Autodesk Inventor part; units mm, degrees
ref_plane "YZ Plane" through (0, 0, 0) normal (1, 0, 0) x (0, 1, 0)
ref_plane "XZ Plane" through (0, 0, 0) normal (0, 1, 0) x (-1, 0, 0)
ref_plane "XY Plane" through (0, 0, 0) normal (0, 0, 1) x (1, 0, 0)
sketch "Boceto6" plane through (0, 0, 0) normal (0, 1, 0) x (-1, 0, 0)
  line L0 (0, 0) -> (100, 0)
  line L1 (100, 0) -> (100, -100)
  line L2 (100, -100) -> (0, -100)
  line L3 (0, -100) -> (0, 0)
  line L4 (97, -97) -> (97, -3)
  line L5 (97, -3) -> (3, -3)
  line L6 (3, -3) -> (3, -97)
  line L7 (3, -97) -> (97, -97)
  line L8 (97, -3) -> (100, -3)
  line L9 (3, -97) -> (3, -106.6251)
  point P0 (3, -100)
  dimension "d46" = 100
  dimension "d47" = 100
  dimension "d48" = 3
extrude "Extrusión6" add sketch "Boceto6" along normal blind 2000 contours L0 L1 L8 L5 L6 L9 L2 L3
sketch "Boceto9" plane through (-100, 0, 0) normal (0, 0, 1) x (1, 0, 0)
  point P0 (100, 0)
sketch "Boceto12" plane through (0, 0, 0) normal (1, 0, 0) x (0, 0, -1)
  line L0 (0, 2000) -> (100, 2000)
  line L1 (100, 0) -> (100, 2000)
  line L2 (0, 2000) -> (100, 2000)
  line L3 (100, 2000) -> (100, 1950)
  line L4 (100, 1950) -> (0, 1950)
  line L5 (0, 1950) -> (0, 2000)
  line L6 (0, 1650) -> (100, 1650)
  line L7 (100, 1650) -> (100, 1600)
  line L8 (100, 1600) -> (0, 1600)
  line L9 (0, 1600) -> (0, 1650)
  line L10 (0, 1300) -> (100, 1300)
  line L11 (100, 1300) -> (100, 1250)
  line L12 (100, 1250) -> (0, 1250)
  line L13 (0, 1250) -> (0, 1300)
  line L14 (0, 950) -> (100, 950)
  line L15 (100, 950) -> (100, 900)
  line L16 (100, 900) -> (0, 900)
  line L17 (0, 900) -> (0, 950)
  line L18 (0, 600) -> (100, 600)
  line L19 (100, 600) -> (100, 550)
  line L20 (100, 550) -> (0, 550)
  line L21 (0, 550) -> (0, 600)
  circle A0 centre (50, 1900) radius 25
  line L22 (0, 0) -> (0, 2000)
  circle A1 centre (50, 1800) radius 25
  circle A2 centre (50, 1700) radius 25
  circle A3 centre (20, 1975) radius 4
  circle A4 centre (45, 1975) radius 4
  circle A5 centre (70, 1975) radius 4
  line L23 (100, 1600) -> (0, 1600)
  line L24 (0, 1650) -> (100, 1650)
  line L25 (100, 1650) -> (100, 1600)
  circle A6 centre (50, 1350) radius 25
  circle A7 centre (50, 1450) radius 25
  circle A8 centre (50, 1550) radius 25
  circle A9 centre (70, 1625) radius 4
  circle A10 centre (45, 1625) radius 4
  circle A11 centre (20, 1625) radius 4
  line L26 (100, 1250) -> (0, 1250)
  line L27 (0, 1300) -> (100, 1300)
  line L28 (100, 1300) -> (100, 1250)
  circle A12 centre (50, 1000) radius 25
  circle A13 centre (50, 1100) radius 25
  circle A14 centre (50, 1200) radius 25
  circle A15 centre (70, 1275) radius 4
  circle A16 centre (45, 1275) radius 4
  circle A17 centre (20, 1275) radius 4
  line L29 (100, 900) -> (0, 900)
  line L30 (0, 950) -> (100, 950)
  line L31 (100, 950) -> (100, 900)
  circle A18 centre (50, 650) radius 25
  circle A19 centre (50, 750) radius 25
  circle A20 centre (50, 850) radius 25
  circle A21 centre (70, 925) radius 4
  circle A22 centre (45, 925) radius 4
  circle A23 centre (20, 925) radius 4
  line L32 (100, 550) -> (0, 550)
  line L33 (0, 600) -> (100, 600)
  line L34 (100, 600) -> (100, 550)
  circle A24 centre (50, 300) radius 25
  circle A25 centre (50, 400) radius 25
  circle A26 centre (50, 500) radius 25
  circle A27 centre (70, 575) radius 4
  circle A28 centre (45, 575) radius 4
  circle A29 centre (20, 575) radius 4
  point P0 (0, 1975)
  point P1 (100, 1975)
  point P2 (100, 1625)
  point P3 (100, 1275)
  point P4 (100, 925)
  point P5 (100, 575)
  dimension "d113" = 50
  dimension "d116" = 350
  dimension "d121" = 50
  dimension "d122" = 50
  dimension "d123" = 50
  dimension "d126" = 100
  dimension "d135" = 8
  dimension "d136" = 8
  dimension "d137" = 8
  dimension "d138" = 25
  dimension "d139" = 25
  dimension "d140" = 25
  dimension "d141" = 20
  dimension "d142" = 30
  dimension "d143" = 25
  dimension "d144" = 25
  dimension "d147" = 350
extrude "Extrusión10" cut sketch "Boceto12" against normal blind 2000 contours A0 | A1 | A2 | A3 | A4 | A5 | A6 | A7 | A8 | A9 | A10 | A11 | A12 | A13 | A14 | A15 | A16 | A17 | A18 | A19 | A20 | A21 | A22 | A23 | A24 | A25 | A26 | A27 | A28 | A29
sketch "Boceto13" plane through (-100, 0, 0) normal (0, 0, 1) x (1, 0, 0)
  line L0 (0, 2000) -> (100, 2000)
  line L1 (100, 694.7481) -> (100, 2000)
  line L2 (0, 2000) -> (100, 2000)
  line L3 (100, 2000) -> (100, 1950)
  line L4 (100, 1950) -> (0, 1950)
  line L5 (0, 1950) -> (0, 2000)
  line L6 (0, 1650) -> (100, 1650)
  line L7 (100, 1650) -> (100, 1600)
  line L8 (100, 1600) -> (0, 1600)
  line L9 (0, 1600) -> (0, 1650)
  line L10 (0, 1300) -> (100, 1300)
  line L11 (100, 1300) -> (100, 1250)
  line L12 (100, 1250) -> (0, 1250)
  line L13 (0, 1250) -> (0, 1300)
  line L14 (0, 950) -> (100, 950)
  line L15 (100, 950) -> (100, 900)
  line L16 (100, 900) -> (0, 900)
  line L17 (0, 900) -> (0, 950)
  line L18 (0, 600) -> (100, 600)
  line L19 (100, 600) -> (100, 550)
  line L20 (100, 550) -> (0, 550)
  line L21 (0, 550) -> (0, 600)
  circle A0 centre (50, 1900) radius 25
  line L22 (0, 692.1927) -> (0, 2000)
  circle A1 centre (50, 1800) radius 25
  circle A2 centre (50, 1700) radius 25
  circle A3 centre (20, 1975) radius 4
  circle A4 centre (45, 1975) radius 4
  circle A5 centre (70, 1975) radius 4
  line L23 (100, 1600) -> (0, 1600)
  line L24 (0, 1650) -> (100, 1650)
  line L25 (100, 1650) -> (100, 1600)
  circle A6 centre (50, 1350) radius 25
  circle A7 centre (50, 1450) radius 25
  circle A8 centre (50, 1550) radius 25
  circle A9 centre (70, 1625) radius 4
  circle A10 centre (45, 1625) radius 4
  circle A11 centre (20, 1625) radius 4
  line L26 (100, 1250) -> (0, 1250)
  line L27 (0, 1300) -> (100, 1300)
  line L28 (100, 1300) -> (100, 1250)
  circle A12 centre (50, 1000) radius 25
  circle A13 centre (50, 1100) radius 25
  circle A14 centre (50, 1200) radius 25
  circle A15 centre (70, 1275) radius 4
  circle A16 centre (45, 1275) radius 4
  circle A17 centre (20, 1275) radius 4
  line L29 (100, 900) -> (0, 900)
  line L30 (0, 950) -> (100, 950)
  line L31 (100, 950) -> (100, 900)
  circle A18 centre (50, 650) radius 25
  circle A19 centre (50, 750) radius 25
  circle A20 centre (50, 850) radius 25
  circle A21 centre (70, 925) radius 4
  circle A22 centre (45, 925) radius 4
  circle A23 centre (20, 925) radius 4
  line L32 (100, 550) -> (0, 550)
  line L33 (0, 600) -> (100, 600)
  line L34 (100, 600) -> (100, 550)
  circle A24 centre (50, 300) radius 25
  circle A25 centre (50, 400) radius 25
  circle A26 centre (50, 500) radius 25
  circle A27 centre (70, 575) radius 4
  circle A28 centre (45, 575) radius 4
  circle A29 centre (20, 575) radius 4
  line L35 (0, 0) -> (0, 2000)
  line L36 (100, 0) -> (100, 2000)
  line L37 (0, 2000) -> (100, 2000)
  point P0 (0, 1975)
  point P1 (100, 1975)
  point P2 (100, 1625)
  point P3 (100, 1275)
  point P4 (100, 925)
  point P5 (100, 575)
  dimension "d166" = 50
  dimension "d167" = 350
  dimension "d168" = 50
  dimension "d169" = 50
  dimension "d170" = 50
  dimension "d171" = 100
  dimension "d172" = 8
  dimension "d173" = 8
  dimension "d174" = 8
  dimension "d175" = 25
  dimension "d176" = 25
  dimension "d177" = 25
  dimension "d178" = 20
  dimension "d179" = 30
  dimension "d180" = 25
  dimension "d181" = 25
  dimension "d182" = 350
  dimension "d186" = 0
  dimension "d187" = 0
  dimension "d188" = 0
extrude "Extrusión11" cut sketch "Boceto13" against normal blind 2000 contours A0 | A1 | A2 | A3 | A4 | A5 | A6 | A7 | A8 | A9 | A10 | A11 | A12 | A13 | A14 | A15 | A16 | A17 | A18 | A19 | A20 | A21 | A22 | A23 | A24 | A25 | A26 | A27 | A28 | A29
properties part number "mesa completa"
Source: CAD feature listing. Evaluate the final solid. Frame: model axes, mm. Round coordinates to 2 decimals unless told otherwise and drop trailing zeros. Loops run counter-clockwise (first coordinate to the right, second up) from the corner with the lowest first, then second, coordinate; pieces in that order, holes last.
(1) Material intervals for probe 1 along X at (y, z) = (1625, -2); probe 2 along Z at (x, y) = (-0.55, 925); probe 3 along X at (y, z) = (1350, -2.3), sorted ascending.
From the geometry:
probe 1: x = -100 to -84, -76 to -59, -51 to -34, -26 to 0
probe 2: z = -100 to -74, -66 to -49, -41 to -24, -16 to 0
probe 3: x = -100 to -75, -25 to 0
(2) Contact query for flat-ended pins moving along their axis: pin 1 Ø10.5 at (x, y) = (-80, 575) entering from -Z; pin 2 Ø5 at (y, z) = (537, -30.5) entering from -X. Output: stop coordinate, or through.
From the geometry:
pin 1: stops at z = -3
pin 2: stops at x = -3
(3) Section query A-A (y = 1800). Output: boundary loops of the cut face in (x, z).
From the geometry:
outline: (-100, -3) - (-75, -3) - (-75, 0) - (-100, 0) - close; (-25, -3) - (-3, -3) - (-3, -25) - (0, -25) - (0, 0) - (-25, 0) - close; (-3, -100) - (0, -100) - (0, -75) - (-3, -75) - close
(4) Pull-direction query (Z, two-part tool) for faces 1 (the cylindrical face through (-53.255, 524.787, -1.479)), 2 (the cylindrical face through (-1.479, 1175.594, -44.58)), 3 (the cylindrical face through (-1.479, 1075.594, -44.58)), 4 (the flat face through (-72, 986, -3)); classes: +Z half, -Z half, draft (parallel to the pull), parting line (faces both ways), or undercut.
From the geometry:
face 1: draft
face 2: undercut
face 3: undercut
face 4: -Z half
(5) Section query B-B (y = 124.5). Output: boundary loops of the cut face in (x, z), and give its area (3 significant figures).
From the geometry:
outline: (-100, -3) - (-3, -3) - (-3, -100) - (0, -100) - (0, 0) - (-100, 0) - close
area: 591 mm2
